from build123d import *

# Parameters (mm, degrees)
BOSS_EXTRUDE1_DEPTH = 3.175
SKETCH2_R           = 1.5
CUT_EXTRUDE1_DEPTH  = 3.175


with BuildPart() as part:
    # Sketch1 → Boss-Extrude1 (new body)
    with BuildSketch(Plane.XY):
        Polygon((40, 279.4), (0, 279.4), (0, 228.6), (-3.175, 228.6), (-3.175, 212.436363636), (0, 212.436363636), (0, 196.272727273), (-3.175, 196.272727273), (-3.175, 180.109090909), (0, 180.109090909), (0, 163.945454545), (-3.175, 163.945454545), (-3.175, 147.781818182), (0, 147.781818182), (0, 131.618181818), (-3.175, 131.618181818), (-3.175, 115.454545455), (0, 115.454545455), (0, 99.290909091), (-3.175, 99.290909091), (-3.175, 83.127272727), (0, 83.127272727), (0, 66.963636364), (-3.175, 66.963636364), (-3.175, 50.8), (0, 50.8), (0, 0), (40, 0), (40, 50.8), (47.35, 50.8), (47.35, 66.963636364), (40, 66.963636364), (40, 83.127272727), (47.35, 83.127272727), (47.35, 99.290909091), (40, 99.290909091), (40, 115.454545455), (47.35, 115.454545455), (47.35, 131.618181818), (40, 131.618181818), (40, 147.781818182), (47.35, 147.781818182), (47.35, 163.945454545), (40, 163.945454545), (40, 180.109090909), (47.35, 180.109090909), (47.35, 196.272727273), (40, 196.272727273), (40, 212.436363636), (47.35, 212.436363636), (47.35, 228.6), (40, 228.6), align=None)
    extrude(amount=BOSS_EXTRUDE1_DEPTH)

    # Sketch2 → Cut-Extrude1 (cut)
    with BuildSketch(Plane.XY.offset(3.175)):
        with Locations((15.875, 20)):
            Circle(SKETCH2_R)
        with Locations((15.875, 35.75)):
            Circle(SKETCH2_R)
        with Locations((15.875, 243.65)):
            Circle(SKETCH2_R)
        with Locations((15.875, 259.4)):
            Circle(SKETCH2_R)
        with Locations((28.3, 20)):
            Circle(SKETCH2_R)
        with Locations((28.3, 35.75)):
            Circle(SKETCH2_R)
        with Locations((28.3, 243.65)):
            Circle(SKETCH2_R)
        with Locations((28.3, 259.4)):
            Circle(SKETCH2_R)
    extrude(amount=-CUT_EXTRUDE1_DEPTH, mode=Mode.SUBTRACT)


solid = part.part
Here's how the part is built. I have some questions about the finished solid (model axes, mm). Coordinates: 2 decimals unless noted, no trailing zeros. Order: outer loops, then holes, each group sorted by start corner. A loop starts at its lowest first (then second) coordinate and runs counter-clockwise, first axis right, second up. Notation, with made-up numbers: (88, 15.5) -> (126, 15.5) arc R22 ccw to (126, 24.5) -> close; hole circle Ø10 at (32, -19.5). An arc over 180 degrees is marked (long way). Answer in a Markdown table with one row per item.
(1) I want a section at C-C on z = 1.25. Count the separate pieces of the cut face and the enclosed holes in it, then the cut area to 3 significant figures.
Answer key:
| item | result |
|---|---|
| separate pieces | 1 |
| enclosed holes | 8 |
| area | 12,100 mm^2 |
(2) I want a section at B-B on y = 204.5. List the corners of the cut face in (x, z) for me (3 decimals), then the cut area to 3 significant figures.
Answer key:
| item | result |
|---|---|
| outline | (0, 0) -> (40, 0) -> (40, 3.175) -> (0, 3.175) -> close |
| area | 127 mm^2 |
(3) I want a section at A-A on x = 44. List the corners of the cut face in (y, z) for me (3 decimals), then the cut area to 3 significant figures.
Answer key:
| item | result |
|---|---|
| outline | (50.8, 0) -> (66.964, 0) -> (66.964, 3.175) -> (50.8, 3.175) -> close; (83.127, 0) -> (99.291, 0) -> (99.291, 3.175) -> (83.127, 3.175) -> close; (115.455, 0) -> (131.618, 0) -> (131.618, 3.175) -> (115.455, 3.175) -> close; (147.782, 0) -> (163.945, 0) -> (163.945, 3.175) -> (147.782, 3.175) -> close; (180.109, 0) -> (196.273, 0) -> (196.273, 3.175) -> (180.109, 3.175) -> close; (212.436, 0) -> (228.6, 0) -> (228.6, 3.175) -> (212.436, 3.175) -> close |
| area | 308 mm^2 |
(4) Will these pins go through, and if not, where does the flat tip stop? pin 1 Ø1 at (x, z) = (-1.5, 1) entering from -Y; pin 2 Ø1 at (x, z) = (-1.5, 1) entering from +Y; pin 3 Ø1.5 at (x, z) = (14, 2.5) entering from -Y; pin 4 Ø1.6 at (y, z) = (172, 1) entering from +X.
Answer key:
| item | result |
|---|---|
| pin 1 | y = 50.8 |
| pin 2 | y = 228.6 |
| pin 3 | y = 0 |
| pin 4 | x = 40 |
(5) Please list where these lines run through material, in increasing order: probe 1 along Y at (x, z) = (28.3, 2.1); probe 2 along Y at (x, z) = (29, 0.5); probe 3 along X at (y, z) = (176.5, 1.3).
Answer key:
| item | result |
|---|---|
| probe 1 | 0 to 18.5, 21.5 to 34.25, 37.25 to 242.15, 245.15 to 257.9, 260.9 to 279.4 |
| probe 2 | 0 to 18.67, 21.33 to 34.42, 37.08 to 242.32, 244.98 to 258.07, 260.73 to 279.4 |
| probe 3 | 0 to 40 |
